Build history of the part. All positions in model axes, mm. A direction names the side the tool comes from. Give positions to 0.01 mm unless a question says otherwise; leave off trailing zeros. Order: outer loops, then holes, each group sorted by start corner. A loop starts at its lowest first (then second) coordinate and runs counter-clockwise, first axis right, second up. Notation, with made-up numbers: (24, 60.5) -> (50, 60.5) arc R15 ccw to (50, 71.5) -> close; hole circle Ø9 at (0.25, 65.25). An arc over 180 degrees is marked (long way). One line per item, written item: value. Start each with the question number.
(1) Saw through at B-B on y = -4. Give the cut face in (x, z), plus the area to 3 significant figures.
(2) Two-plate mould, pull along Y, no slides. Class faces 4 (the cylindrical face through (1.08, -4.61, -7.26)), 5 (the cylindrical face through (-4.618, 9.374, 12.424)), 6 (the cylindrical face through (1.409, 6.345, -0.139)), 7 (the cylindrical face through (4.912, 9.374, -12.496)): +Y half, -Y half, draft (parallel to the pull), parting line (faces both ways), or undercut.
(3) Which spindle directions (+Z, -Z, +X, -X, +Y, -Y) get a long thin tool onto all of the face, cutting with end or side? Do faces 1 (the cylindrical face through (10.1, 7.7, 12.4)), 2 (the flat face through (3, -6, 9.92)), 3 (the cylindrical face through (-0.15, -7.67, 11.34)). Say none if no direction does.
(4) Probe line 1 (Z direction, x = -8.5, y = -4.75); line 2 (Y direction, x = -9.53, z = 12.95); line 3 (Z direction, x = 0.75, y = -7). List the from-to ranges inside material, lowest first.
(5) Saw through at A-A on x = 0. Count the separate pieces of the cut face and the enclosed holes in it, plus the area to 3 significant figures.
(6) Saw through at D-D on z = -12.46. Give the cut face in (x, y) (3 decimals).
(7) Saw through at C-C on x = 9. Give the cut face in (y, z), plus the area to 3 significant figures.
(8) Pin check, flat tips, straight feed: pin 1 (1 mm diameter, centred on y = -5.5, z = -0.5, fed in from +X); pin 2 (3 mm diameter, centred on x = 0, z = -6.92, fed in from +Y); pin 3 (3.5 mm diameter, centred on x = 0, z = 6.92, fed in from -Y). Stop position of each tip, or through.
```python
from build123d import *

# Parameters (mm, degrees)
CROQUIS3_R                  = 3
CORTAR_EXTRUIR1_DEPTH       = 35.96541148
TALADRO_ROSCADO_4_403_D     = 2.2606
TALADRO_ROSCADO_4_403_DEPTH = 5.08
TALADRO_ROSCADO_4_405_D     = 2.2606
TALADRO_ROSCADO_4_405_DEPTH = 8.87
TALADRO_ROSCADO_4_405_TIP   = 0.679152758
TALADRO_ROSCADO_4_404_D     = 2.2606
TALADRO_ROSCADO_4_404_DEPTH = 12.699
TALADRO_ROSCADO_4_404_TIP   = 0.679152758


with BuildPart() as part:
    # Croquis2 → Revolución1 (revolve)
    with BuildSketch(Plane(origin=(0, 0, 0), x_dir=(0, 0, -1), z_dir=(1, 0, 0)), mode=Mode.PRIVATE) as revoluci_n1_sk:
        Polygon((-9.92, 6.5), (9.92, 6.5), (9.92, 12.7), (15, 12.7), (15, 0), (-15, 0), (-15, 12.7), (-9.92, 12.7), align=None)
    revolve(revoluci_n1_sk.sketch.rotate(Axis((0, 0, -15), (0, 0, 1)), 90), axis=Axis((0, 0, -15), (0, 0, 1)))

    # Croquis3 → Cortar-Extruir1 (cut, through all)
    with BuildSketch(Plane.XY.offset(15)):
        Circle(CROQUIS3_R)
    extrude(amount=-CORTAR_EXTRUIR1_DEPTH, mode=Mode.SUBTRACT)

    # Taladro roscado #4-403
    with Locations(Plane.XY.offset(-9.92)):
        with Locations((-9.53, 0), (-4.765, 8.253222098), (4.765, 8.253222098), (9.53, 0), (4.765, -8.253222098), (-4.765, -8.253222098), (0, 0)):
            Hole(TALADRO_ROSCADO_4_403_D / 2, depth=TALADRO_ROSCADO_4_403_DEPTH)

    # Taladro roscado #4-405
    with Locations(Plane.XY.offset(15)):
        with Locations((-9.53, 0), (-4.765, 8.253222098), (4.765, 8.253222098), (9.53, 0), (4.765, -8.253222098), (-4.765, -8.253222098)):
            Hole(TALADRO_ROSCADO_4_405_D / 2, depth=TALADRO_ROSCADO_4_405_DEPTH)
            with Locations((0, 0, -(TALADRO_ROSCADO_4_405_DEPTH + TALADRO_ROSCADO_4_405_TIP / 2))):  # 118° drill point
                Cone(0, TALADRO_ROSCADO_4_405_D / 2, TALADRO_ROSCADO_4_405_TIP, mode=Mode.SUBTRACT)

    # Taladro roscado #4-404
    with Locations(Plane(origin=(0, -12.7, 0), x_dir=(-1, 0, 0), z_dir=(0, -1, 0))):
        with Locations((0, 12.46), (0, 6.92), (0, -6.92), (0, -12.46)):
            Hole(TALADRO_ROSCADO_4_404_D / 2, depth=TALADRO_ROSCADO_4_404_DEPTH)
            with Locations((0, 0, -(TALADRO_ROSCADO_4_404_DEPTH + TALADRO_ROSCADO_4_404_TIP / 2))):  # 118° drill point
                Cone(0, TALADRO_ROSCADO_4_404_D / 2, TALADRO_ROSCADO_4_404_TIP, mode=Mode.SUBTRACT)


solid = part.part
```
Results below:
1. outline: (-12.05, -15) -> (12.05, -15) -> (12.05, -9.92) -> (5.12, -9.92) -> (5.12, 9.92) -> (12.05, 9.92) -> (12.05, 15) -> (-12.05, 15) -> (-12.05, 9.92) -> (-5.12, 9.92) -> (-5.12, -9.92) -> (-12.05, -9.92) -> close; hole circle Ø2.26 at (0, -12.46); hole circle Ø2.26 at (0, -6.92); hole circle Ø2.26 at (0, 6.92); hole circle Ø2.26 at (0, 12.46)
1. area: 432 mm²
2. face 4: draft
2. face 5: undercut
2. face 6: parting line
2. face 7: undercut
3. face 1: +Z, -Z
3. face 2: none
3. face 3: -Y
4. line 1: z = -15 to -9.92, 9.92 to 15
4. line 2: y = -8.39 to -1.13, 1.13 to 8.39
4. line 3: z = -15 to -13.31, -11.61 to -9.92, 9.92 to 11.61, 13.31 to 15
5. separate pieces: 6
5. enclosed holes: 0
5. area: 276 mm²
6. outline: (-1.13, -12.65) -> (-1.13, -2.779) arc R3 cw (long way) to (1.13, -2.779) -> (1.13, -12.65) arc R12.7 ccw (long way) to start; hole circle Ø2.261 at (-9.53, 0); hole circle Ø2.261 at (-4.765, -8.253); hole circle Ø2.261 at (-4.765, 8.253); hole circle Ø2.261 at (4.765, -8.253); hole circle Ø2.261 at (4.765, 8.253); hole circle Ø2.261 at (9.53, 0)
7. outline: (-8.96, -15) -> (-1, -15) -> (-1, -9.92) -> (-8.96, -9.92) -> close; (-8.96, 9.92) -> (-1, 9.92) -> (-1, 15) -> (-8.96, 15) -> close; (1, -15) -> (8.96, -15) -> (8.96, -9.92) -> (1, -9.92) -> close; (1, 9.92) -> (8.96, 9.92) -> (8.96, 15) -> (1, 15) -> close
7. area: 162 mm²
8. pin 1: stops at x = 4.15
8. pin 2: stops at y = 6.5
8. pin 3: stops at y = -6.5
